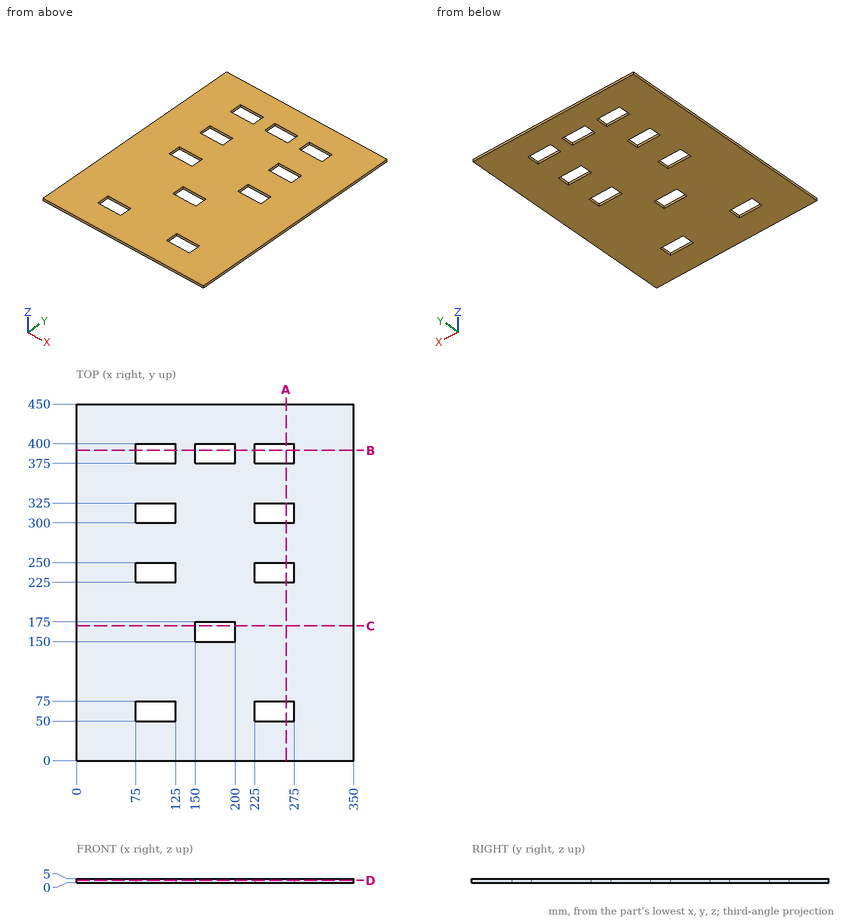
For this review, use the dimensioned drawing (mm, ordinates from the lowest corner) and the shaded views. Give positions to 0.01 mm unless a question says otherwise; leave off trailing zeros. Loops run counter-clockwise (first coordinate to the right, second up) from the corner with the lowest first, then second, coordinate; pieces in that order, holes last.
Item 1: Take a section at A-A, the plane x = 264.5. State the section outline as (y, z) points.
Item 2: For line 1 along Y through (x, z) = (255, 3.7); line 2 along Y through (x, z) = (152.5, 1.4); line 3 along X through (y, z) = (154, 3.3), list the stretches that pass through material, from the lowest coordinate up.
Item 3: Take a section at C-C, the plane y = 170. State the section outline as (x, z) points.
Item 4: Take a section at D-D, the plane z = 2.75. Give the number of separate pieces and of enclosed holes in the cut face, and give its area (3 significant figures).
Item 5: Take a section at B-B, the plane y = 391.5. State the section outline as (x, z) points, and give its area (3 significant figures).
Calculated:
1. outline: (0, 0) - (50, 0) - (50, 5) - (0, 5) - close; (75, 0) - (225, 0) - (225, 5) - (75, 5) - close; (250, 0) - (300, 0) - (300, 5) - (250, 5) - close; (325, 0) - (375, 0) - (375, 5) - (325, 5) - close; (400, 0) - (450, 0) - (450, 5) - (400, 5) - close
2. line 1: y = 0 to 50, 75 to 225, 250 to 300, 325 to 375, 400 to 450
2. line 2: y = 0 to 150, 175 to 375, 400 to 450
2. line 3: x = 0 to 150, 200 to 350
3. outline: (0, 0) - (150, 0) - (150, 5) - (0, 5) - close; (200, 0) - (350, 0) - (350, 5) - (200, 5) - close
4. separate pieces: 1
4. enclosed holes: 10
4. area: 145,000 mm2
5. outline: (0, 0) - (75, 0) - (75, 5) - (0, 5) - close; (125, 0) - (150, 0) - (150, 5) - (125, 5) - close; (200, 0) - (225, 0) - (225, 5) - (200, 5) - close; (275, 0) - (350, 0) - (350, 5) - (275, 5) - close
5. area: 1,000 mm2
